Here's how the part is built. I have some questions about the finished solid (model axes, mm). Face numbers are marked on the shaded views. A direction names the side the tool comes from. Give positions to 0.01 mm unless a question says otherwise; leave off trailing zeros. Loops run counter-clockwise (first coordinate to the right, second up) from the corner with the lowest first, then second, coordinate; pieces in that order, holes last. Notation, with made-up numbers: (43, 40) - (67, 40) arc R27 cw to (67, 63) - close; hole circle Ø7 at (46, 63.25). An arc over 180 degrees is marked (long way). Put each result on its own line as item: value. Start each with the question number.
from build123d import *

# Parameters (mm, degrees)
SKETCH_1_W          = 24.91
SKETCH_1_H          = 17.95
EXTRUDE_1_DEPTH     = 7.65
CUT_EXTRUDE_1_DEPTH = 5.26
SKETCH_3_R          = 5.48
EXTRUDE_2_DEPTH     = 7.65
SKETCH_4_W          = 24.91
SKETCH_4_H          = 17.95
EXTRUDE_3_DEPTH     = 2.41


with BuildPart() as part:
    # 草图1 → 凸台-拉伸1 (new body)
    with BuildSketch(Plane.XY):
        Rectangle(SKETCH_1_W, SKETCH_1_H)
    extrude(amount=EXTRUDE_1_DEPTH)

    # 草图2 → 切除-拉伸1 (cut)
    with BuildSketch(Plane(origin=(0, 0, 0), x_dir=(-1, 0, 0), z_dir=(0, 0, -1))):
        with BuildLine():
            Line((-7.56, -8.975), (-7.56, -7.872967992))
            ThreePointArc((-7.56, -7.872967992), (-10.915, 0), (-7.56, 7.872967992))
            Line((-7.56, 7.872967992), (-7.56, 8.975))
            Line((-7.56, 8.975), (7.56, 8.975))
            Line((7.56, 8.975), (7.56, 7.872967992))
            ThreePointArc((7.56, 7.872967992), (10.915, 0), (7.56, -7.872967992))
            Line((7.56, -7.872967992), (7.56, -8.975))
            Line((7.56, -8.975), (-7.56, -8.975))
        make_face()
    extrude(amount=-CUT_EXTRUDE_1_DEPTH, mode=Mode.SUBTRACT)

    # 草图3 → 凸台-拉伸2 (add)
    with BuildSketch(Plane.XY.offset(7.65)):
        Circle(SKETCH_3_R)
    extrude(amount=-EXTRUDE_2_DEPTH)

    # 草图4 → 凸台-拉伸3 (add)
    with BuildSketch(Plane.XY):
        Rectangle(SKETCH_4_W, SKETCH_4_H)
    extrude(amount=-EXTRUDE_3_DEPTH)


solid = part.part
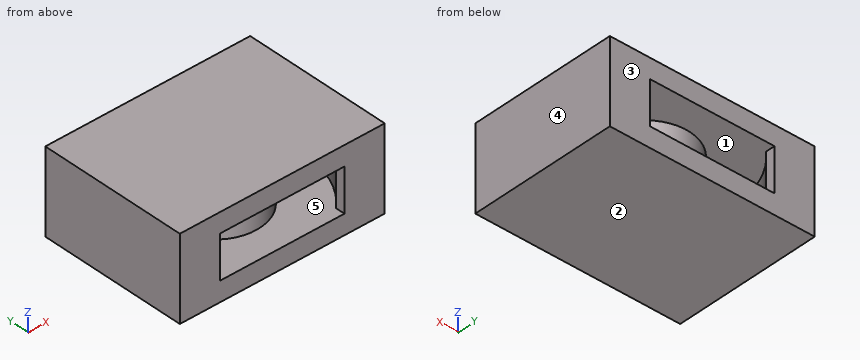
1) I need wall thicknesses on line 1 (Z direction, x = -6.75, y = 5); line 2 (X direction, y = 2.75, z = 1.5) (3 decimals); line 3 (X direction, y = -0.5, z = 3) (3 decimals). Which ranges of each line are inside material? Lowest first, please.
2) Suppose I cut it at A-A on z = 3. Please give me the cut outline in (x, y) (3 decimals), plus the area to 3 significant figures.
3) Suppose I cut it at D-D on y = 7. Please give me the cut outline in (x, z) (3 decimals).
4) Thinking about a two-plate mould opening in Y: for the marked faces 1, 2 and 3, which applies, pulls with the +Y half, pulls with the -Y half, needs draft (parallel to the pull), parting line crosses it, or undercut?
5) Suppose I cut it at C-C on y = 0. Please give me the cut outline in (x, z) (3 decimals), plus the area to 3 significant figures.
6) Suppose I cut it at B-B on x = 0. Please give me the cut outline in (y, z) (3 decimals), plus the area to 3 significant figures.
7) Which directions (+Z, -Z, +X, -X, +Y, -Y) give clear straight access to the entire face, cutting with the end or side of a thin tool? Please do the marked faces 4 and 5.
Ans:
1. line 1: z = -2.41 to 0, 5.26 to 7.65
1. line 2: x = -12.455 to -10.563, -4.74 to 4.74, 10.563 to 12.455
1. line 3: x = -12.455 to -10.904, -5.457 to 5.457, 10.904 to 12.455
2. outline: (-12.455, -8.975) - (-7.56, -8.975) - (-7.56, -7.873) arc R10.915 cw to (-7.56, 7.873) - (-7.56, 8.975) - (-12.455, 8.975) - close; circle Ø10.96 at (0, 0); (7.56, -8.975) - (12.455, -8.975) - (12.455, 8.975) - (7.56, 8.975) - (7.56, 7.873) arc R10.915 cw to (7.56, -7.873) - close
2. area: 197 mm²
3. outline: (-12.455, -2.41) - (12.455, -2.41) - (12.455, 7.65) - (-12.455, 7.65) - close; hole (-8.375, 0) - (8.375, 0) - (8.375, 5.26) - (-8.375, 5.26) - close
4. face 1: undercut
4. face 2: needs draft
4. face 3: pulls with the +Y half
5. outline: (-12.455, -2.41) - (12.455, -2.41) - (12.455, 7.65) - (-12.455, 7.65) - close; hole (-10.915, 0) - (-5.48, 0) - (-5.48, 5.26) - (-10.915, 5.26) - close; hole (5.48, 0) - (10.915, 0) - (10.915, 5.26) - (5.48, 5.26) - close
5. area: 193 mm²
6. outline: (-8.975, -2.41) - (8.975, -2.41) - (8.975, 0) - (5.48, 0) - (5.48, 5.26) - (8.975, 5.26) - (8.975, 7.65) - (-8.975, 7.65) - (-8.975, 5.26) - (-5.48, 5.26) - (-5.48, 0) - (-8.975, 0) - close
6. area: 144 mm²
7. face 4: +Z, -Z, +X, +Y, -Y
7. face 5: none
